Verification items for the finished model (mm, model axes). A direction names the side the tool comes from. Round coordinates to 2 decimals unless told otherwise and drop trailing zeros. Loops run counter-clockwise (first coordinate to the right, second up) from the corner with the lowest first, then second, coordinate; pieces in that order, holes last. Notation, with made-up numbers: (20, 49) - (59, 49) arc R11 ccw to (59, 55) - close; hole circle Ø11 at (15.5, 59.5). An arc over 180 degrees is marked (long way). Use CSV: the item, a comma, the result in double quotes.
Autodesk Inventor part; units mm, degrees
ref_plane "YZ Plane" through (0, 0, 0) normal (1, 0, 0) x (0, 1, 0)
ref_plane "XZ Plane" through (0, 0, 0) normal (0, 1, 0) x (-1, 0, 0)
ref_plane "XY Plane" through (0, 0, 0) normal (0, 0, 1) x (1, 0, 0)
sketch "Эскиз2" plane through (0, 0, 0) normal (0, 0, 1) x (1, 0, 0)
  circle A0 centre (0, 0) radius 36.5
  circle A1 centre (0, 0) radius 32.0179
  dimension "d2" = 73
extrude "Выдавливание1" add sketch "Эскиз2" along normal blind 15 contours A0 | A1
draft "НаклГрань1" angle 4.5 pull direction (0, 0, 1) faces at (36.3902, -2.8285, 10) fixed edges at (-36.5, 0, 0)
shell "Оболочка1" thickness 2 removed faces 1 at (4.5012, 0.5261, 0)
sketch "Эскиз3" plane through (0, 0, 15) normal (0, 0, 1) x (1, 0, 0)
  circle A0 centre (0, 0) radius 30.3888
extrude "Выдавливание2" add sketch "Эскиз3" along normal blind 3
properties part number "CUP"
1) Access from +Z, -Z, +X, -X, +Y, -Y to the whole of each face (thin tool, end or side, straight path). Record for faces 4 (the face through (0, 0, 18)), 5 (the face through (15.53, 26.33, 15)), 6 (the face through (0, 0, 13)).
Returned:
face 4,"+Z, +X, -X, +Y, -Y"
face 5,"+Z"
face 6,"-Z"
2) Cross-section at D-D, the plane z = 16.5. Record the cut outline in (x, y).
Returned:
outline,"circle Ø60.78 at (0, 0)"
3) Thickness scan on probe 1 along Z at (x, y) = (-14, 23.5); probe 2 along Y at (x, z) = (-27, 9); probe 3 along Y at (x, z) = (-23, 8.5). Record the ranges inside material, lowest first. Write a range as [from, to].
Returned:
probe 1,"z = [13, 18]"
probe 2,"y = [-23.5, -20.31], [20.31, 23.5]"
probe 3,"y = [-27.47, -24.8], [24.8, 27.47]"
4) Cross-section at C-C, the plane z = 10.5. Record the cut outline in (x, y), then the cut area to 3 significant figures.
Returned:
outline,"circle Ø71.35 at (0, 0); hole circle Ø67.33 at (0, 0)"
area,"437 mm²"
5) Mould release check, pull along Y, two halves, no side actions. Record for faces 1 (the face through (-33.73, -1.48, 9.3)), 2 (the face through (27, 22, 0)), 3 (the face through (-7.729, 34.808, 10.728)): +Y half, -Y half, draft (parallel to the pull), parting line (faces both ways), or undercut.
Returned:
face 1,"undercut"
face 2,"draft"
face 3,"parting line"
6) Cross-section at A-A, the plane x = 0. Record the cut outline in (y, z), then the cut area to 3 significant figures.
Returned:
outline,"(-36.5, 0) - (-34.49, 0) - (-33.47, 13) - (33.47, 13) - (34.49, 0) - (36.5, 0) - (35.32, 15) - (30.39, 15) - (30.39, 18) - (-30.39, 18) - (-30.39, 15) - (-35.32, 15) - close"
area,"376 mm²"
7) Gauge pin test, flat ends, axial feed: pin 1 Ø5 at (x, z) = (-24.5, 11.5) entering from +Y; pin 2 Ø1.5 at (x, z) = (-29, 7) entering from +Y; pin 3 Ø5 at (y, z) = (-6, 12.5) entering from +X. Record the tip position at first contact, or that the pin passes through.
Returned:
pin 1,"stops at y = 28"
pin 2,"stops at y = 22.24"
pin 3,"stops at x = 35.41"
